Build history of the part. All positions in model axes, mm. Face numbers are marked on the shaded views. A direction names the side the tool comes from. Round coordinates to 2 decimals unless told otherwise and drop trailing zeros. Loops run counter-clockwise (first coordinate to the right, second up) from the corner with the lowest first, then second, coordinate; pieces in that order, holes last. Notation, with made-up numbers: (89.5, -23.5) - (135.5, -23.5) arc R18 cw to (135.5, -11.5) - close; hole circle Ø4 at (82, -38). An arc over 180 degrees is marked (long way). Use a Markdown table: item, result.
Autodesk Inventor part; units mm, degrees
ref_plane "YZ Plane" through (0, 0, 0) normal (1, 0, 0) x (0, 1, 0)
ref_plane "XZ Plane" through (0, 0, 0) normal (0, 1, 0) x (-1, 0, 0)
ref_plane "XY Plane" through (0, 0, 0) normal (0, 0, 1) x (1, 0, 0)
sketch "Sketch1" plane through (0, 0, 0) normal (1, 0, 0) x (0, 1, 0)
  line L0 (0, 0) -> (60, 0)
  line L1 (60, 0) -> (60, 20)
  line L2 (60, 20) -> (0, 20)
  line L3 (0, 20) -> (0, 0)
  line L4 (60, 10) -> (0, 10) construction
  line L5 (60, 10) -> (30, 10) construction
  line L6 (30, 10) -> (0, 10) construction
  circle A0 centre (45, 10) radius 2.75
  circle A1 centre (15, 10) radius 2.75
  dimension "d0" = 60
  dimension "d1" = 20
  dimension "d2" = 5.5
  dimension "d3" = 5.5
extrude "Extrusion1" add sketch "Sketch1" against normal blind 6
sketch "Sketch2" plane through (-6, 0, 0) normal (-1, 0, 0) x (0, 0, 1)
  circle A0 centre (10, 45) radius 2.75
  circle A1 centre (10, 15) radius 2.75
  circle A2 centre (10, 45) radius 6.25
  circle A3 centre (10, 15) radius 6.25
  line L0 (20, 60) -> (0, 60)
  line L1 (12, 60) -> (12, 0)
  line L2 (8, 60) -> (8, 0)
  line L3 (0, 0) -> (20, 0)
  line L4 (0, 60) -> (0, 0)
  line L5 (20, 0) -> (20, 60)
  line L6 (12, 56.5) -> (17, 56.5)
  line L7 (17, 56.5) -> (17, 60)
  line L8 (8, 56.5) -> (3, 56.5)
  line L9 (3, 56.5) -> (3, 60)
  line L10 (8, 3.5) -> (3, 3.5)
  line L11 (3, 3.5) -> (3, 0)
  line L12 (12, 3.5) -> (17, 3.5)
  line L13 (17, 3.5) -> (17, 0)
  point P0 (12, 39.0786)
  point P1 (12, 50.9214)
  point P2 (8, 50.9214)
  point P3 (8, 39.0786)
  point P4 (8, 20.9214)
  point P5 (8, 9.0786)
  point P6 (12, 9.0786)
  point P7 (12, 20.9214)
  dimension "d6" = 3.5
  dimension "d7" = 8
  dimension "d8" = 8
  dimension "d9" = 3.5
  dimension "d10" = 3.5
  dimension "d11" = 3.5
  dimension "d16" = 3.5
extrude "Extrusion2" add sketch "Sketch2" along normal blind 22.1 contours A0 L1 A2 | A0 L2 A2 L1 | L1 A2 L2 A0 | A0 L2 A2 | A2 L2 L0 L1 | L1 A3 L2 A2 | L1 L0 L7 L6 | L1 A1 L2 A3 | A3 L1 A1 | L8 L9 L0 L2 | L2 A1 A3 | L2 A1 L1 A3 | A3 L1 L3 L2 | L2 L3 L11 L10 | L12 L13 L3 L1
sketch "Sketch3" plane through (-28.1, 0, 0) normal (-1, 0, 0) x (0, 0, 1)
  circle A0 centre (10, 45) radius 2.75
  circle A1 centre (10, 15) radius 2.75
  line L0 (20, 0) -> (20, 60)
  line L1 (17, 0) -> (20, 0)
  line L2 (3, 0) -> (17, 0)
  line L3 (0, 0) -> (3, 0)
  line L4 (0, 60) -> (0, 0)
  line L5 (3, 60) -> (0, 60)
  line L6 (17, 60) -> (3, 60)
  line L7 (20, 60) -> (17, 60)
extrude "Extrusion3" add sketch "Sketch3" along normal blind 6
equation "\"d3\" = d2"
equation "\"d16\" = d6"
properties part number "X Axis Belt and V Wheel Plate Spacer"
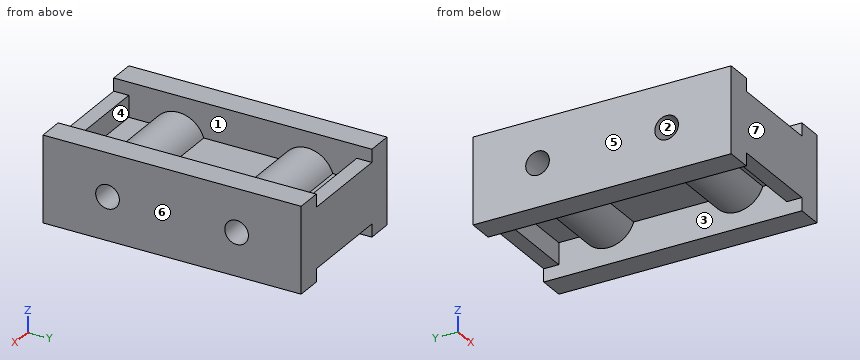
Q1. Cut at C-C, the plane y = 27.5. List the corners of the cut face in (x, z).
Results found:
| item | result |
|---|---|
| outline | (-34.1, 0) - (-28.1, 0) - (-28.1, 8) - (-6, 8) - (-6, 0) - (0, 0) - (0, 20) - (-6, 20) - (-6, 12) - (-28.1, 12) - (-28.1, 20) - (-34.1, 20) - close |
Q2. Pull direction X, two halves, no side cores. Call the marked faces 4, 5, 6 and 7: pulls with the +X half, pulls with the -X half, needs draft (parallel to the pull), parting line crosses it, or undercut.
Results found:
| item | result |
|---|---|
| face 4 | undercut |
| face 5 | pulls with the -X half |
| face 6 | pulls with the +X half |
| face 7 | needs draft |
Q3. Probe line 1 (Y direction, x = -11.5, z = 10); line 2 (Y direction, x = -4, z = 9); line 3 (X direction, y = 27, z = 16). List the from-to ranges inside material, lowest first.
Results found:
| item | result |
|---|---|
| line 1 | y = 0 to 12.25, 17.75 to 42.25, 47.75 to 60 |
| line 2 | y = 0 to 12.44, 17.56 to 42.44, 47.56 to 60 |
| line 3 | x = -34.1 to -28.1, -6 to 0 |
Q4. Cut at A-A, the plane x = -11.5. List the corners of the cut face in (y, z), plus the area to 3 significant figures.
Results found:
| item | result |
|---|---|
| outline | (0, 3) - (3.5, 3) - (3.5, 8) - (9.08, 8) arc R6.25 ccw to (20.92, 8) - (39.08, 8) arc R6.25 ccw to (50.92, 8) - (56.5, 8) - (56.5, 3) - (60, 3) - (60, 17) - (56.5, 17) - (56.5, 12) - (50.92, 12) arc R6.25 ccw to (39.08, 12) - (20.92, 12) arc R6.25 ccw to (9.08, 12) - (3.5, 12) - (3.5, 17) - (0, 17) - close; hole circle Ø5.5 at (15, 10); hole circle Ø5.5 at (45, 10) |
| area | 410 mm2 |
Q5. Cut at B-B, the plane z = 5. List the corners of the cut face in (x, y), plus the area to 3 significant figures.
Results found:
| item | result |
|---|---|
| outline | (-34.1, 0) - (0, 0) - (0, 60) - (-34.1, 60) - close; hole (-28.1, 3.5) - (-6, 3.5) - (-6, 11.25) - (-28.1, 11.25) - close; hole (-28.1, 18.75) - (-6, 18.75) - (-6, 41.25) - (-28.1, 41.25) - close; hole (-28.1, 48.75) - (-6, 48.75) - (-6, 56.5) - (-28.1, 56.5) - close |
| area | 1,210 mm2 |
Q6. Cut at D-D, the plane z = 9. List the corners of the cut face in (x, y).
Results found:
| item | result |
|---|---|
| outline | (-34.1, 0) - (0, 0) - (0, 12.44) - (-34.1, 12.44) - close; (-34.1, 17.56) - (0, 17.56) - (0, 42.44) - (-34.1, 42.44) - close; (-34.1, 47.56) - (0, 47.56) - (0, 60) - (-34.1, 60) - close |
Q7. Which spindle directions (+Z, -Z, +X, -X, +Y, -Y) get a long thin tool onto all of the face, cutting with end or side? Do the marked faces 1, 2 and 3. Say none if no direction does.
Results found:
| item | result |
|---|---|
| face 1 | +Z |
| face 2 | +X, -X |
| face 3 | -Z |
Q8. Drop flat-ended pins along their axis: pin 1 (4.5 mm diameter, centred on x = -16.5, y = 53.5, fed in from -Z); pin 2 (9 mm diameter, centred on x = -18.5, y = 31, fed in from +Z); pin 3 (10 mm diameter, centred on x = -13.5, y = 9.5, fed in from +Z). Give the stop position or say it passes through.
Results found:
| item | result |
|---|---|
| pin 1 | stops at z = 8 |
| pin 2 | stops at z = 12 |
| pin 3 | stops at z = 16.23 |
